```python
from build123d import *

# Parameters (mm, degrees)
CROQUIS1_R              = 30
SALIENTE_EXTRUIR1_DEPTH = 12
CROQUIS2_R              = 4
CROQUIS3_R              = 6.125
SALIENTE_EXTRUIR2_DEPTH = 10
CROQUIS4_R              = 1.25
CORTAR_EXTRUIR1_DEPTH   = 45.09081537
CHAFL_N1_SIZE           = 3
CROQUIS5_R              = 4


with BuildPart() as part:
    # Croquis1 → Saliente-Extruir1 (new body)
    with BuildSketch(Plane.XY):
        Circle(CROQUIS1_R)
    extrude(amount=SALIENTE_EXTRUIR1_DEPTH)

    # Croquis2 → Cortar-Revolución1 (revolve, cut)
    with BuildSketch(Plane(origin=(0, 0, 0), x_dir=(1, 0, 0), z_dir=(0, 1, 0))):
        with Locations((-30, -6)):
            Circle(CROQUIS2_R)
    revolve(axis=Axis((0, 0, 0), (0, 0, 1)), mode=Mode.SUBTRACT)

    # Croquis3 → Saliente-Extruir2 (add)
    with BuildSketch(Plane.XY.offset(12)):
        Circle(CROQUIS3_R)
        with BuildLine():
            Line((-2.125, 1.936491673), (-2.125, -1.936491673))
            ThreePointArc((-2.125, -1.936491673), (0, -2.875), (2.125, -1.936491673))
            Line((2.125, -1.936491673), (2.125, 1.936491673))
            ThreePointArc((2.125, 1.936491673), (0, 2.875), (-2.125, 1.936491673))
        make_face(mode=Mode.SUBTRACT)
    extrude(amount=SALIENTE_EXTRUIR2_DEPTH)

    # Croquis4 → Cortar-Extruir1 (cut, through all)
    with BuildSketch(Plane.XY.offset(12)):
        Circle(CROQUIS4_R)
    extrude(amount=-CORTAR_EXTRUIR1_DEPTH, mode=Mode.SUBTRACT)

    # Chaflán1
    chafl_n1_edges = [part.edges().sort_by_distance(p)[0] for p in [
        (-6.125, 0, 12),
    ]]
    chamfer(chafl_n1_edges, length=CHAFL_N1_SIZE)

    # Croquis5 → Revolución1 (revolve)
    with BuildSketch(Plane(origin=(0, 0, 0), x_dir=(0, 0, -1), z_dir=(1, 0, 0)), mode=Mode.PRIVATE) as revoluci_n1_sk:
        with Locations((-6, 30)):
            Circle(CROQUIS5_R)
    revolve(revoluci_n1_sk.sketch.rotate(Axis((0, 0, 0), (0, 0, -1)), 270), axis=Axis((0, 0, 0), (0, 0, -1)))


solid = part.part
```
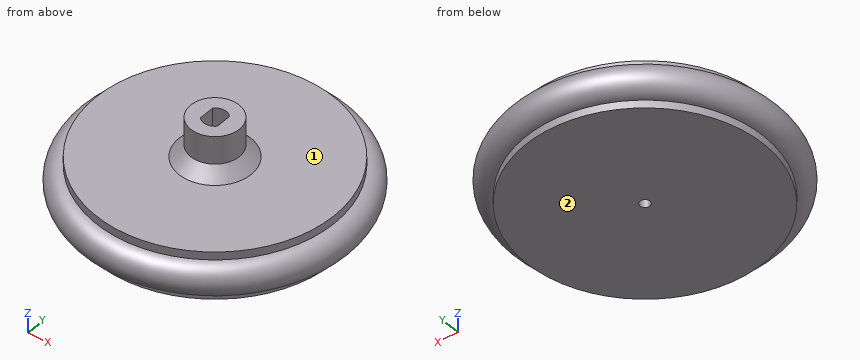
Geometry: final body of the model. Coordinates: model frame, mm. Face numbers are marked on the shaded views. A direction names the side the tool comes from. Round coordinates to 2 decimals unless told otherwise and drop trailing zeros. Order: outer loops, then holes, each group sorted by start corner. A loop starts at its lowest first (then second) coordinate and runs counter-clockwise, first axis right, second up. Notation, with made-up numbers: (49.25, -12) - (71.25, -12) arc R22 ccw to (71.25, -5) - close; hole circle Ø1 at (-19.5, 84). An arc over 180 degrees is marked (long way). Write item = value, one per line. Start each with the question number.
Q1. Access query for the marked faces 1 and 2. Directions: +Z, -Z, +X, -X, +Y, -Y. A direction counts if a zero-diameter tool reaches every point of the face in a straight line with its end or side. Return the directions, or none.
Q2. Cut plane B-B on y = 0. Return the cut outline in (x, z) (3 decimals).
Q3. Cut plane A-A on x = 0. Return the cut outline in (y, z) (3 decimals).
Q4. Ray query, line 1 (Y direction, x = 0, z = 6); line 2 (Y direction, x = 0, z = 3.25); line 3 (Z direction, x = -15, y = 16.5). Return the intervals inside material, ascending. Write a range as from..to.
Q5. Pin query (flat end, axial travel): pin 1 (1.5 mm diameter, centred on y = 6.5, z = 4, fed in from +X); pin 2 (1.9 mm diameter, centred on y = 0.5, z = 16.5, fed in from -X) (3 decimals); pin 3 (2 mm diameter, centred on y = 0.5, z = 18.5, fed in from +X) (3 decimals); pin 4 (6 mm diameter, centred on x = -12, z = 16.5, fed in from -Y). Return the tip coordinate at first contact, or that it passes through.
Outcome:
q1.face_1 = +Z
q1.face_2 = -Z, +X, -X, +Y, -Y
q2.outline = (-30, 0) - (-1.25, 0) - (-1.25, 12) - (-2.125, 12) - (-2.125, 22) - (-6.125, 22) - (-6.125, 15) - (-9.125, 12) - (-30, 12) - (-30, 10) arc R4 ccw to (-30, 2) - close; (1.25, 0) - (30, 0) - (30, 2) arc R4 ccw to (30, 10) - (30, 12) - (9.125, 12) - (6.125, 15) - (6.125, 22) - (2.125, 22) - (2.125, 12) - (1.25, 12) - close
q3.outline = (-30, 0) - (-1.25, 0) - (-1.25, 12) - (-2.875, 12) - (-2.875, 22) - (-6.125, 22) - (-6.125, 15) - (-9.125, 12) - (-30, 12) - (-30, 10) arc R4 ccw to (-30, 2) - close; (1.25, 0) - (30, 0) - (30, 2) arc R4 ccw to (30, 10) - (30, 12) - (9.125, 12) - (6.125, 15) - (6.125, 22) - (2.875, 22) - (2.875, 12) - (1.25, 12) - close
q4.line_1 = -34..-1.25, 1.25..34
q4.line_2 = -32.9..-1.25, 1.25..32.9
q4.line_3 = 0..12
q5.pin_1 = 33.21
q5.pin_2 = -6.125
q5.pin_3 = 6.125
q5.pin_4 = through
